Read the model definition and answer for the solid it produces. Units are mm, in the model's axes. A direction names the side the tool comes from. Give positions to 0.01 mm unless a question says otherwise; leave off trailing zeros. Loops run counter-clockwise (first coordinate to the right, second up) from the corner with the lowest first, then second, coordinate; pieces in that order, holes last. Notation, with made-up numbers: (23, 84) - (34, 84) arc R33 ccw to (34, 112) - close; hole circle Ø9 at (57, 78.25). An arc over 180 degrees is marked (long way). Write item = value, one per line.
Autodesk Inventor part; units mm, degrees
ref_plane "YZ Plane" through (0, 0, 0) normal (1, 0, 0) x (0, 1, 0)
ref_plane "XZ Plane" through (0, 0, 0) normal (0, 1, 0) x (-1, 0, 0)
ref_plane "XY Plane" through (0, 0, 0) normal (0, 0, 1) x (1, 0, 0)
sketch "スケッチ1" plane through (0, 0, 0) normal (0, 1, 0) x (-1, 0, 0)
  line L0 (-3, 0.3) -> (-3, 3.7)
  line L1 (-3.3, 4) -> (-3.7, 4)
  line L2 (-4, 3) -> (-4, 1)
  line L3 (-4, 1) -> (-6, 1)
  line L4 (-6, 1) -> (-6, 0)
  line L5 (-6, 0) -> (-3.3, 0)
  line L6 (-3, 3.7) -> (-3.3, 4)
  line L7 (-3, 0.3) -> (-3.3, 0)
  line L8 (-3.7, 4) -> (-4, 3)
  line L9 (0, -0.8) -> (0, 4.8)
  point P0 (0, 0)
  point P1 (-3, 0)
  point P2 (-3, 4)
  point P3 (-4, 4)
  dimension "d2" = 1
  dimension "d9" = 1
  dimension "d11" = 6
  dimension "d12" = 8
  dimension "d13" = 12
  dimension "d14" = 0.3
  dimension "d15" = 0.3
  dimension "d16" = 0.3
  dimension "d17" = 0.3
  dimension "d18" = 0.3
  dimension "d19" = 4
revolve "回転1" add sketch "スケッチ1" angle 360 about axis through (0, 0, -10) along (0, 0, 1)
sketch "스케치2" plane through (0, 0, 0) normal (0, 0, -1) x (-1, 0, 0)
  circle A0 centre (0, 0) radius 3.3
  circle A1 centre (0, 0) radius 6
  circle A2 centre (0, 0) radius 3.025
  dimension "d20" = 6.05
extrude "돌출1" cut sketch "스케치2" against normal up to surface (4 mm away) contours A2
sketch "스케치3" plane through (0, 0, 0) normal (0, 0, -1) x (-1, 0, 0)
  circle A0 centre (0, 0) radius 3.3
  circle A1 centre (0, 0) radius 6
  circle A2 centre (0, 0) radius 5
  dimension "d23" = 10
extrude "돌출2" cut sketch "스케치3" against normal through all contours A1
sketch "스케치4" plane through (0, 0, 4) normal (0, 0, 1) x (1, 0, 0)
  circle A0 centre (0, 0) radius 4
  circle A1 centre (0, 0) radius 3.7
  circle A2 centre (0, 0) radius 2.5
  dimension "d26" = 5
extrude "돌출3" add sketch "스케치4" against normal up to surface (4 mm away) contours A0 | A1
sketch "스케치5" plane through (0, 0, 4) normal (0, 0, 1) x (1, 0, 0)
  circle A0 centre (0, 0) radius 3.5
  circle A1 centre (0, 0) radius 4
  circle A2 centre (0, 0) radius 2.5
  dimension "d29" = 7
extrude "돌출4" cut sketch "스케치5" against normal up to surface (3 mm away) contours A1
chamfer "모따기1" distance 0.275 angle 45 1 edges at (-3.5, 0, 4)
chamfer "모따기2" distance 0.275 angle 45 2 edges at (-2.5, 0, 4) (-2.5, 0, 0)
equation "\"d15\" = d14"
equation "\"d16\" = d14"
equation "\"d17\" = d16"
equation "\"d18\" = d14"
properties part number "80F-0503"
1) A tool of negligible diameter and unlimited length cuts with its end or side. For faces 1 (the face through (3.233, -1.341, 2.382)), 2 (the face through (2.2, -2.2, 0)), from which of +Z, -Z, +X, -X, +Y, -Y can it reach the whole face along a straight path? Write none if from no direction.
Output:
face_1 = +Z
face_2 = -Z, +X, -X, +Y, -Y
2) This flat-tipped pin is pushed along its axis until it touches: P1, Ø2, axis at y = -2, z = 1, coming from the +X side. Where does it stop, or does it pass through?
Output:
P1 = 4.9
3) Find the intervals of material crossed by probe 1 along Y at (x, z) = (0, 1.15); probe 2 along X at (y, z) = (-0.75, 0.7); probe 3 along X at (y, z) = (0.25, 2.45), in increasing order.
Output:
probe_1 = -3.5 to -2.5, 2.5 to 3.5
probe_2 = -4.94 to -2.38, 2.38 to 4.94
probe_3 = -3.49 to -2.49, 2.49 to 3.49
4) A cutting plane is placed at D-D on x = 4. Determine the outline of the cut face in (y, z).
Output:
outline = (-3, 0) - (3, 0) - (3, 1) - (-3, 1) - close
5) The mould has two halves that part along Y. Classify faces 3 (the face through (1.08, -4.88, 0.49)), 4 (the face through (-0.54, -2.44, 2.02)), 5 (the face through (2.2, -3.3, 1)): pulls with the +Y half, pulls with the -Y half, needs draft (parallel to the pull), parting line crosses it, or undercut.
Output:
face_3 = parting line crosses it
face_4 = undercut
face_5 = needs draft
6) A cutting plane is placed at A-A on y = 0. Determine the outline of the cut face in (x, z) (3 decimals).
Output:
outline = (-5, 0) - (-2.775, 0) - (-2.5, 0.275) - (-2.5, 3.725) - (-2.775, 4) - (-3.225, 4) - (-3.5, 3.725) - (-3.5, 1) - (-5, 1) - close; (2.5, 0.275) - (2.775, 0) - (5, 0) - (5, 1) - (3.5, 1) - (3.5, 3.725) - (3.225, 4) - (2.775, 4) - (2.5, 3.725) - close
7) A cutting plane is placed at C-C on z = 2.15. Determine the outline of the cut face in (x, y).
Output:
outline = circle Ø7 at (0, 0); hole circle Ø5 at (0, 0)
